from build123d import *

# Parameters (mm, degrees)
SKETCH1_R             = 22.5
BOSS_EXTRUDE1_DEPTH   = 19
BOSS_EXTRUDE1_2_DEPTH = 19
BOSS_EXTRUDE2_DEPTH   = 9
CUT_EXTRUDE1_DEPTH    = 4
SKETCH6_W             = 94
SKETCH6_H             = 30
BOSS_EXTRUDE3_DEPTH   = 9
SKETCH4_R             = 12.5
CUT_EXTRUDE2_DEPTH    = 39
SKETCH5_R             = 4.5
CUT_EXTRUDE3_DEPTH    = 224.7
CUT_EXTRUDE4_DEPTH    = 224.7


with BuildPart() as part:
    # Sketch1 → Boss-Extrude1 (new body, symmetric)
    with BuildSketch(Plane.XY):
        Circle(SKETCH1_R)
    extrude(amount=BOSS_EXTRUDE1_DEPTH, both=True)



with BuildPart() as body_2:
    # Sketch1 → Boss-Extrude1 2 (new body, symmetric)
    with BuildSketch(Plane.XY):
        with BuildLine():
            Line((-36, -201.2), (36, -201.2))
            ThreePointArc((36, -201.2), (0, -165.2), (-36, -201.2))
        make_face()
    extrude(amount=BOSS_EXTRUDE1_2_DEPTH, both=True)


with BuildPart() as part_1:
    add(part.part)

    add(body_2.part)  # Boss-Extrude2 merges body 2
    # Sketch2 → Boss-Extrude2 (add, symmetric)
    with BuildSketch(Plane.XY):
        with BuildLine():
            Line((-16.279722223, -152.158712146), (-10, -32.334474052))
            ThreePointArc((-10, -32.334474052), (-11.381584619, -23.310643729), (-16.234582266, -15.578457518))
            ThreePointArc((-16.234582266, -15.578457518), (0, -22.5), (16.234582266, -15.578457518))
            ThreePointArc((16.234582266, -15.578457518), (11.381584619, -23.310643729), (10, -32.334474052))
            Line((10, -32.334474052), (16.279722223, -152.158712146))
            ThreePointArc((16.279722223, -152.158712146), (19.307974883, -165.464636648), (26.63284908, -176.978287635))
            ThreePointArc((26.63284908, -176.978287635), (0, -165.2), (-26.63284908, -176.978287635))
            ThreePointArc((-26.63284908, -176.978287635), (-19.307974883, -165.464636648), (-16.279722223, -152.158712146))
        make_face()
    extrude(amount=BOSS_EXTRUDE2_DEPTH, both=True)

    # Sketch3 → Cut-Extrude1 (cut)
    with BuildSketch(Plane.XY.offset(9)):
        with BuildLine():
            Line((-8, -145.6), (-8, -55.6))
            ThreePointArc((-8, -55.6), (0, -47.6), (8, -55.6))
            Line((8, -55.6), (8, -145.6))
            ThreePointArc((8, -145.6), (0, -153.6), (-8, -145.6))
        make_face()
    cut_extrude1 = extrude(amount=-CUT_EXTRUDE1_DEPTH, mode=Mode.SUBTRACT)

    # Mirror1: Cut-Extrude1 across plane
    add(cut_extrude1.mirror(Plane.XY), mode=Mode.SUBTRACT)

    # Sketch6 → Boss-Extrude3 (add, symmetric)
    with BuildSketch(Plane.XY):
        with Locations((0, -186.2)):
            Rectangle(SKETCH6_W, SKETCH6_H)
    extrude(amount=BOSS_EXTRUDE3_DEPTH, both=True)

    # Sketch4 → Cut-Extrude2 (cut, through all)
    with BuildSketch(Plane.XY.offset(19)):
        Circle(SKETCH4_R)
        with BuildLine():
            Line((-27, -201.2), (27, -201.2))
            ThreePointArc((27, -201.2), (0, -174.2), (-27, -201.2))
        make_face()
    extrude(amount=-CUT_EXTRUDE2_DEPTH, mode=Mode.SUBTRACT)

    # Sketch5 → Cut-Extrude3 (cut, through all)
    with BuildSketch(Plane.XZ.offset(201.2)):
        with Locations((-38, 0)):
            Circle(SKETCH5_R)
        with Locations((38, 0)):
            Circle(SKETCH5_R)
    extrude(amount=-CUT_EXTRUDE3_DEPTH, mode=Mode.SUBTRACT)

    # Sketch7 → Cut-Extrude4 (cut, through all)
    with BuildSketch(Plane.XZ.offset(201.2)):
        with BuildLine():
            ThreePointArc((-38, -9), (-44.363961031, -6.363961031), (-47, 0))
            Line((-47, 0), (-47, -9))
            Line((-47, -9), (-38, -9))
        make_face()
        with BuildLine():
            Line((-38, 9), (-47, 9))
            Line((-47, 9), (-47, 0))
            ThreePointArc((-47, 0), (-44.363961031, 6.363961031), (-38, 9))
        make_face()
    cut_extrude4 = extrude(amount=-CUT_EXTRUDE4_DEPTH, mode=Mode.SUBTRACT)

    # Mirror2: Cut-Extrude4 across plane
    add(cut_extrude4.mirror(Plane(origin=(0, 0, 0), x_dir=(0, 0, 1), z_dir=(1, 0, 0))), mode=Mode.SUBTRACT)


solid = part_1.part
CAD build for the part. Positions are in the model's coordinates, mm. A direction names the side the tool comes from. Coordinates: 2 decimals unless noted, no trailing zeros. Order: outer loops, then holes, each group sorted by start corner. A loop starts at its lowest first (then second) coordinate and runs counter-clockwise, first axis right, second up.
Item 1: Two-plate mould, pull along X, no slides. Class faces 4 (the face through (-8, -101, 7)), 5 (the face through (0.79, -165.21, 14.07)), 6 (the face through (-33, -201.2, 0)), 7 (the face through (-13.184, -93.085, 0.126)): +X half, -X half, draft (parallel to the pull), parting line (faces both ways), or undercut.
Check sheet entries:
face 4: undercut
face 5: parting line
face 6: draft
face 7: -X half
Item 2: 3-axis set-ups, long thin cutter, end or side, ignore diameter. For faces 1 (the face through (-0.176, -47.602, 7.028)), 2 (the face through (18.02, -161.92, 0.13)), 3 (the face through (0.176, -153.598, -7.028)): which of +Z, -Z, +X, -X, +Y, -Y reach the whole face in a straight line?
Check sheet entries:
face 1: +Z
face 2: +Z, -Z, +X
face 3: -Z
Item 3: Band-saw the part on A-A on z = -12. List the corners of the cut face in (x, y), plus the area to 3 significant figures.
Check sheet entries:
outline: (-36, -201.2) - (-27, -201.2) arc R27 cw to (27, -201.2) - (36, -201.2) arc R36 ccw to start; circle Ø45 at (0, 0); hole circle Ø25 at (0, 0)
area: 1,990 mm2
Item 4: Band-saw the part on B-B on y = 0. List the corners of the cut face in (x, z).
Check sheet entries:
outline: (-22.5, -19) - (-12.5, -19) - (-12.5, 19) - (-22.5, 19) - close; (12.5, -19) - (22.5, -19) - (22.5, 19) - (12.5, 19) - close
Item 5: Pin check, flat tips, straight feed: pin 1 Ø13 at (x, y) = (2.5, -88) entering from -Z; pin 2 Ø4 at (x, z) = (-1, 9.5) entering from -Y; pin 3 Ø22.5 at (x, y) = (0, 0) entering from -Z; pin 4 Ø13 at (x, y) = (2, -125) entering from +Z. Stop position of each tip, or through.
Check sheet entries:
pin 1: stops at z = -9
pin 2: stops at y = -174.37
pin 3: passes through
pin 4: stops at z = 9
Item 6: Band-saw the part on D-D on y = -103. List the corners of the cut face in (x, z), plus the area to 3 significant figures.
Check sheet entries:
outline: (-13.7, -9) - (-8, -9) - (-8, -5) - (8, -5) - (8, -9) - (13.7, -9) - (13.7, 9) - (8, 9) - (8, 5) - (-8, 5) - (-8, 9) - (-13.7, 9) - close
area: 365 mm2
Item 7: Band-saw the part on C-C on z = 7. List the corners of the cut face in (x, y).
Check sheet entries:
outline: (-43.66, -201.2) - (-27, -201.2) arc R27 cw to (27, -201.2) - (43.66, -201.2) - (43.66, -171.2) - (22.26, -171.2) arc R40 cw to (16.28, -152.16) - (10, -32.33) arc R22.5 cw to (16.23, -15.58) arc R22.5 ccw (long way) to (-16.23, -15.58) arc R22.5 cw to (-10, -32.33) - (-16.28, -152.16) arc R40 cw to (-22.26, -171.2) - (-43.66, -171.2) - close; hole circle Ø25 at (0, 0); hole (-8, -145.6) arc R8 ccw to (8, -145.6) - (8, -55.6) arc R8 ccw to (-8, -55.6) - close
Item 8: Drill centre lines: L1, parallel to Y at x = 5.5, z = 6.5; L2, parallel to Z at x = -38, y = -187; L3, parallel to Y at x = 0, z = -4.5. Where is each one in solid material? Low to high.
Check sheet entries:
L1: y = -174.77 to -151.41, -49.79 to -11.22, 11.22 to 21.82
L2: z = -9 to -4.5, 4.5 to 9
L3: y = -174.2 to -12.5, 12.5 to 22.5
